Here's how the part is built. I have some questions about the finished solid (model axes, mm). Face numbers are marked on the shaded views. A direction names the side the tool comes from. Round coordinates to 2 decimals unless told otherwise and drop trailing zeros. Write each loop counter-clockwise with the first axis right and the second up, starting at its lowest first coordinate (ties: lowest second). Pieces come first, ordered by that corner, then holes. Notation, with made-up numbers: (30.25, -5) - (74.25, -5) arc R19 ccw to (74.25, 30) - close; hole circle Ø11 at (82.5, 79.25). An arc over 180 degrees is marked (long way). Write item = value, one per line. Start each with the question number.
Item 1: If we section it at C-C (x = 1.5): Please give me the cut outline in (y, z), and give its area (3 significant figures).
Item 2: If we section it at A-A (z = 8.75): Please give me the cut outline in (x, y), and give its area (3 significant figures).
Item 3: For P1, Ø6.5, axis at x = -2.5, y = -5.5, coming from the +Z side, with a flat end and sliding along its axis, tell me the tip position at first contact or that it passes through.
Item 4: Thinking about a two-plate mould opening in X: for the marked faces 1, 2 and 3, which applies, pulls with the +X half, pulls with the -X half, needs draft (parallel to the pull), parting line crosses it, or undercut?
Item 5: Which directions (+Z, -Z, +X, -X, +Y, -Y) give clear straight access to the entire face, cutting with the end or side of a thin tool? Please do the marked faces 4 and 5.
Item 6: If I drill on line 1 along X through (y, z) = (-33, 2.5); line 2 along Z through (x, y) = (-3, 19), over which ranges is the centre line in solid material (lowest first)? Write a range as [from, to].
Item 7: If we section it at B-B (y = 1): Please give me the cut outline in (x, z), and give its area (3 significant figures).
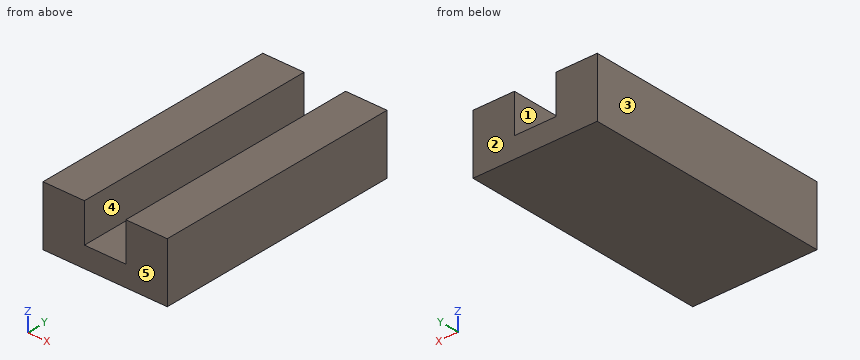
```python
from build123d import *

# Parameters (mm, degrees)
F0_W     = 38.1762
F0_H     = 76.2
F1_DEPTH = 6.35
F2_W     = 12.7254
F2_H     = 76.2
F3_DEPTH = 11.938
F4_DEPTH = 11.938


with BuildPart() as f1:
    # F0 (on Top) → F1 (new body)
    with BuildSketch(Plane.XY):
        Rectangle(F0_W, F0_H)
    extrude(amount=-F1_DEPTH)

    # F2 (on face) → F3 (join)
    with BuildSketch(Plane.XY):
        with Locations((-12.7254, 0)):
            Rectangle(F2_W, F2_H)
    extrude(amount=F3_DEPTH)

    # F2 (on face) → F4 (join)
    with BuildSketch(Plane.XY):
        with Locations((12.7254, 0)):
            Rectangle(F2_W, F2_H)
    extrude(amount=F4_DEPTH)


solid = f1.part
```
Reply:
q1.outline = (-38.1, -6.35) - (38.1, -6.35) - (38.1, 0) - (-38.1, 0) - close
q1.area = 484 mm2
q2.outline = (-19.09, -38.1) - (-6.36, -38.1) - (-6.36, 38.1) - (-19.09, 38.1) - close; (6.36, -38.1) - (19.09, -38.1) - (19.09, 38.1) - (6.36, 38.1) - close
q2.area = 1,940 mm2
q3.P1 = 0
q4.face_1 = undercut
q4.face_2 = needs draft
q4.face_3 = pulls with the -X half
q5.face_4 = +Z, +Y, -Y
q5.face_5 = +Z, -Z, +X, -X, -Y
q6.line_1 = [-19.09, -6.36], [6.36, 19.09]
q6.line_2 = [-6.35, 0]
q7.outline = (-19.09, -6.35) - (19.09, -6.35) - (19.09, 11.94) - (6.36, 11.94) - (6.36, 0) - (-6.36, 0) - (-6.36, 11.94) - (-19.09, 11.94) - close
q7.area = 546 mm2
